Build history of the part. All positions in model axes, mm. Face numbers are marked on the shaded views. Give positions to 0.01 mm unless a question says otherwise; leave off trailing zeros. Order: outer loops, then holes, each group sorted by start corner. A loop starts at its lowest first (then second) coordinate and runs counter-clockwise, first axis right, second up. Notation, with made-up numbers: (15.25, 76) - (72.25, 76) arc R15 cw to (72.25, 88) - close; hole circle Ø3 at (57.5, 31.25). An arc over 180 degrees is marked (long way). Write each question's results on one line, items separated by ' | '. Start each with the question number.
1) Cut at D-D on x = 0. List the corners of the cut face in (y, z).
2) Drill centre lines: line 1 along X through (y, z) = (9.75, -19.05); line 2 along X through (y, z) = (15, -19.05); line 3 along X through (y, z) = (10.5, -13). Where is each one in solid material? Low to high. Write a range as from..to.
3) Cut at C-C on z = -19.05. State how many separate pieces and enclosed holes the cut face has, plus the area to 3 significant figures.
4) Drop flat-ended pins along their axis: pin 1 Ø1.2 at (x, z) = (-13.5, -18.5) entering from +Y; pin 2 Ø1.2 at (x, z) = (-4.5, -16.5) entering from +Y; pin 3 Ø1.2 at (x, z) = (9.5, -12) entering from +Y. Give the stop position or say it passes through.
5) Two-plate mould, pull along X, no slides. Class the marked faces 1, 2 and 3: +X half, -X half, draft (parallel to the pull), parting line (faces both ways), or undercut.
6) Cut at A-A on x = -31.75. List the corners of the cut face in (y, z).
7) Cut at B-B on y = 5.5. List the corners of the cut face in (x, z), plus the area to 3 significant figures.
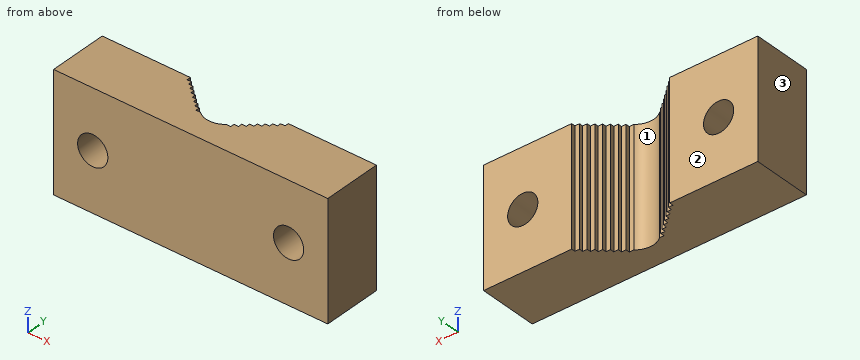
from build123d import *

# Parameters (mm, degrees)
SKETCH1_W               = 88.9
SKETCH1_H               = 19.05
BOSS_EXTRUDE1_DEPTH     = 38.1
CUT_EXTRUDE1_REACH      = 40.1
F_3_8_CLEARANCE_HOLE1_D = 9.8044


with BuildPart() as part:
    # Sketch1 → Boss-Extrude1 (new body)
    with BuildSketch(Plane.XY):
        with Locations((0, 9.525)):
            Rectangle(SKETCH1_W, SKETCH1_H)
    extrude(amount=-BOSS_EXTRUDE1_DEPTH)

    # Sketch2 → Cut-Extrude1 (cut, up to next)
    with BuildSketch(Plane.XY, mode=Mode.PRIVATE) as cut_extrude1_sk1:
        with BuildLine():
            Line((-15.875, 19.05), (0, 19.05))
            Line((0, 19.05), (15.875, 19.05))
            Line((15.875, 19.05), (15.875, 17.78))
            Line((15.875, 17.78), (14.410694861, 17.78))
            Line((14.410694861, 17.78), (14.410694861, 16.51))
            Line((14.410694861, 16.51), (12.946389723, 16.51))
            Line((12.946389723, 16.51), (12.946389723, 15.24))
            Line((12.946389723, 15.24), (11.482084584, 15.24))
            Line((11.482084584, 15.24), (11.482084584, 13.97))
            Line((11.482084584, 13.97), (10.017779445, 13.97))
            Line((10.017779445, 13.97), (10.017779445, 12.7))
            Line((10.017779445, 12.7), (8.553474306, 12.7))
            Line((8.553474306, 12.7), (8.553474306, 11.43))
            Line((8.553474306, 11.43), (7.089169168, 11.43))
            Line((7.089169168, 11.43), (7.089169168, 10.16))
            Line((7.089169168, 10.16), (5.624864029, 10.16))
            Line((5.624864029, 10.16), (5.624864029, 8.89))
            Line((5.624864029, 8.89), (4.16055889, 8.89))
            ThreePointArc((4.16055889, 8.89), (0, 7.337108475), (-4.16055889, 8.89))
            Line((-4.16055889, 8.89), (-5.624864029, 8.89))
            Line((-5.624864029, 8.89), (-5.624864029, 10.16))
            Line((-5.624864029, 10.16), (-7.089169168, 10.16))
            Line((-7.089169168, 10.16), (-7.089169168, 11.43))
            Line((-7.089169168, 11.43), (-8.553474306, 11.43))
            Line((-8.553474306, 11.43), (-8.553474306, 12.7))
            Line((-8.553474306, 12.7), (-10.017779445, 12.7))
            Line((-10.017779445, 12.7), (-10.017779445, 13.97))
            Line((-10.017779445, 13.97), (-11.482084584, 13.97))
            Line((-11.482084584, 13.97), (-11.482084584, 15.24))
            Line((-11.482084584, 15.24), (-12.946389723, 15.24))
            Line((-12.946389723, 15.24), (-12.946389723, 16.51))
            Line((-12.946389723, 16.51), (-14.410694861, 16.51))
            Line((-14.410694861, 16.51), (-14.410694861, 17.78))
            Line((-14.410694861, 17.78), (-15.875, 17.78))
            Line((-15.875, 17.78), (-15.875, 19.05))
        make_face()
    cut_extrude1_tool1 = extrude(cut_extrude1_sk1.sketch, amount=-CUT_EXTRUDE1_REACH, mode=Mode.PRIVATE) & part.part
    add(cut_extrude1_tool1.solids().sort_by_distance((0, 14.620592, 0))[0], mode=Mode.SUBTRACT)

    # 3/8 Clearance Hole1 (through all)
    with Locations(Plane(origin=(0, 19.05, 0), x_dir=(1, 0, 0), z_dir=(0, 1, 0))):
        with Locations((-31.75, 19.05), (31.75, 19.05)):
            Hole(F_3_8_CLEARANCE_HOLE1_D / 2)


solid = part.part
Results:
1) outline: (0, -38.1) - (7.34, -38.1) - (7.34, 0) - (0, 0) - close
2) line 1: -44.45..-36.65, -26.85..-5.62, 5.62..26.85, 36.65..44.45 | line 2: -44.45..-36.65, -26.85..-11.48, 11.48..26.85, 36.65..44.45 | line 3: -44.45..-7.09, 7.09..44.45
3) separate pieces: 3 | enclosed holes: 0 | area: 1,090 mm^2
4) pin 1: y = 16.51 | pin 2: y = 8.89 | pin 3: y = 13.97
5) face 1: undercut | face 2: draft | face 3: -X half
6) outline: (0, -38.1) - (19.05, -38.1) - (19.05, -23.95) - (0, -23.95) - close; (0, -14.15) - (19.05, -14.15) - (19.05, 0) - (0, 0) - close
7) outline: (-44.45, -38.1) - (44.45, -38.1) - (44.45, 0) - (-44.45, 0) - close; hole circle Ø9.8 at (-31.75, -19.05); hole circle Ø9.8 at (31.75, -19.05) | area: 3,240 mm^2
